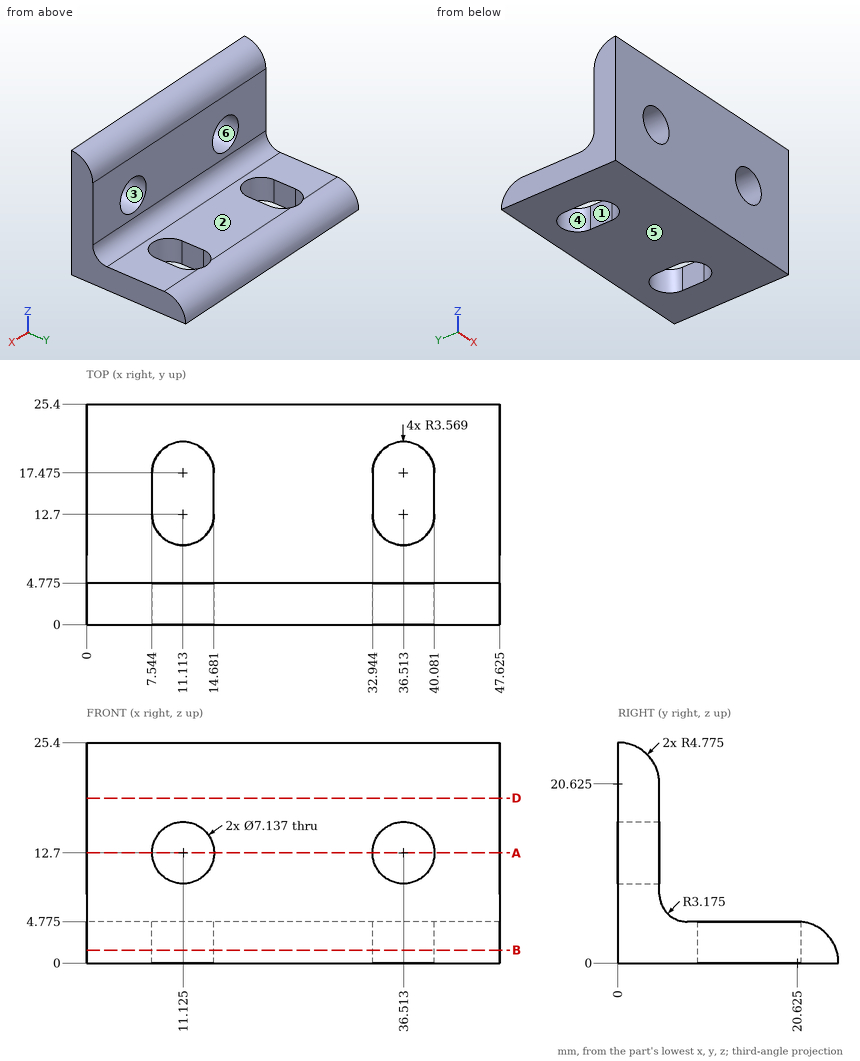
Print and shaded views of the part. All mm, measured from the part's lowest x, y and z. A direction names the side the tool comes from. Give positions to 0.01 mm unless a question says otherwise; leave off trailing zeros. Loops run counter-clockwise (first coordinate to the right, second up) from the corner with the lowest first, then second, coordinate; pieces in that order, holes last. Notation, with made-up numbers: (-32, 61) -> (-23, 61) arc R17 ccw to (-23, 72) -> close; hole circle Ø10 at (82.25, -12.75). An arc over 180 degrees is marked (long way). One line per question, with ' | ' between items. Start each with the question number.
1) 3-axis set-ups, long thin cutter, end or side, ignore diameter. For the marked faces 1, 2 and 3: which of +Z, -Z, +X, -X, +Y, -Y reach the whole face in a straight line?
2) Probe L1, parallel to X at y = 1.4, z = 12.7 (1 decimal); L2, parallel to X at y = 13.5, z = 4.5 (1 decimal); L3, parallel to Y at x = 25, z = 16.5 (1 decimal). List the from-to ranges inside material, lowest first.
3) Cut at B-B (z = 1.5). Give the cut face in (x, y) (1 decimal).
4) Cut at A-A (z = 12.7). Give the cut face in (x, y) (1 decimal).
5) Two-plate mould, pull along Z, no slides. Class the marked faces 4, 5 and 6: released by +Z, released by -Z, zero draft, split by the parting line, or undercut.
6) Cut at D-D (z = 19). Give the cut face in (x, y) (1 decimal).
7) Pin check, flat tips, straight feed: pin 1 (6.5 mm diameter, centred on x = 11.13, z = 12.7, fed in from -Y); pin 2 (5 mm diameter, centred on x = 6, y = 4, fed in from +Z); pin 3 (14 mm diameter, centred on x = 17, y = 14.5, fed in from +Z); pin 4 (4 mm diameter, centred on x = 14.5, z = 14.5, fed in from +Y) (1 decimal). Stop position of each tip, or through.
Return value:
1) face 1: +Z, -Z | face 2: +Z, +X, -X, +Y | face 3: +Y, -Y
2) L1: 0 to 7.6, 14.7 to 32.9, 40.1 to 47.6 | L2: 0 to 7.5, 14.7 to 32.9, 40.1 to 47.6 | L3: 0 to 4.8
3) outline: (0, 0) -> (47.6, 0) -> (47.6, 25.2) -> (0, 25.2) -> close; hole (7.5, 12.7) arc R3.6 ccw to (14.7, 12.7) -> (14.7, 17.5) arc R3.6 ccw to (7.5, 17.5) -> close; hole (32.9, 12.7) arc R3.6 ccw to (40.1, 12.7) -> (40.1, 17.5) arc R3.6 ccw to (32.9, 17.5) -> close
4) outline: (0, 0) -> (7.6, 0) -> (7.6, 4.8) -> (0, 4.8) -> close; (14.7, 0) -> (32.9, 0) -> (32.9, 4.8) -> (14.7, 4.8) -> close; (40.1, 0) -> (47.6, 0) -> (47.6, 4.8) -> (40.1, 4.8) -> close
5) face 4: zero draft | face 5: released by -Z | face 6: undercut
6) outline: (0, 0) -> (47.6, 0) -> (47.6, 4.8) -> (0, 4.8) -> close
7) pin 1: through | pin 2: z = 25.16 | pin 3: z = 4.81 | pin 4: y = 4.8
